Verification items for this drawing (mm, ordinates from the low corner). A direction names the side the tool comes from. Give positions to 0.01 mm unless a question says otherwise; leave off trailing zeros. Write each loop counter-clockwise with the first axis right and the second up, starting at its lowest first coordinate (ties: lowest second). Pieces come first, ordered by that corner, then holes. Notation, with made-up numbers: (-13.5, 15.25) -> (-1.5, 15.25) arc R38 ccw to (-1.5, 54.25) -> close; hole circle Ø4 at (82.25, 12). An arc over 180 degrees is marked (long way). One line per item, written item: value.
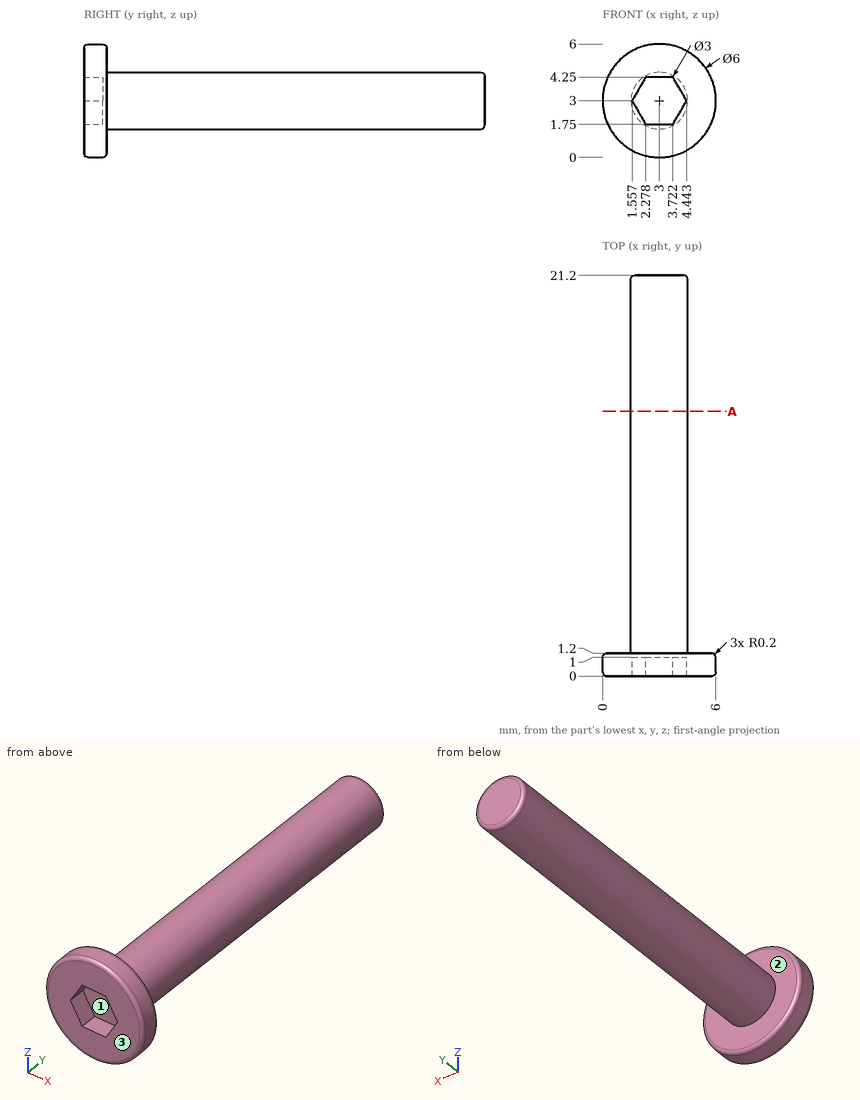
1) Scan lines: probe 1 along Y at (x, z) = (2.75, 5); probe 2 along Z at (x, y) = (1.75, 11.5); probe 3 along Z at (x, y) = (3.5, 8) (1 decimal). Record each from-to range of solid material in increasing order.
Verdict:
probe 1: 0 to 1.2
probe 2: 2.17 to 3.83
probe 3: 1.6 to 4.4
2) Depth check by flat-ended pin: pin 1 Ø0.7 at (x, z) = (2.5, 3.5) entering from -Y; pin 2 Ø3 at (x, y) = (3, 8) entering from +Z; pin 3 Ø1.5 at (y, z) = (10, 0.5) entering from -X. Enter the tip coordinate at first touch or a pass-through.
Verdict:
pin 1: y = 1
pin 2: z = 4.5
pin 3: through
3) Tool access check on the marked faces 1, 2 and 3. Record the directions out of +Z, -Z, +X, -X, +Y, -Y that give a thin tool (end or side, any length) a straight path to the whole face; none if there is none.
Verdict:
face 1: -Y
face 2: +Y
face 3: +Z, -Z, +X, -X, -Y
4) Sectioned sample at A-A on y = 14. Record the cut outline in (x, z).
Verdict:
outline: circle Ø3 at (3, 3)
